For this review, take the finished solid that the model builds, in its own axes (mm). Face numbers are marked on the shaded views. Round coordinates to 2 decimals unless told otherwise and drop trailing zeros. Write each loop counter-clockwise with the first axis right and the second up, starting at its lowest first coordinate (ties: lowest second). Pieces come first, ordered by that corner, then holes. Notation, with made-up numbers: M -37,62 L 10,62 A15 cw 10,68 Z; hole C 5,31 d2. An arc over 180 degrees is marked long. Answer in a Markdown table with one row per item.
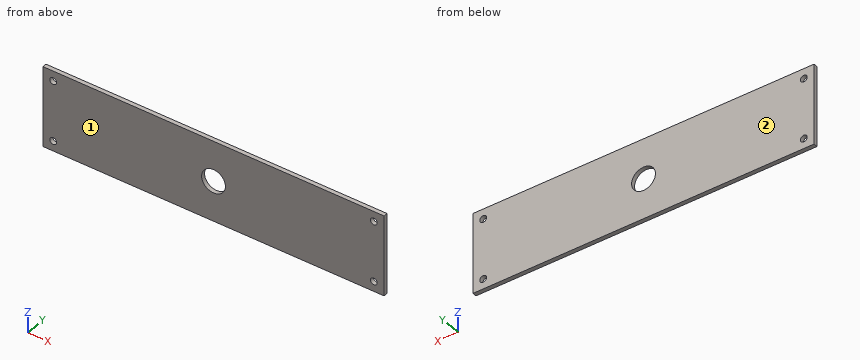
```python
from build123d import *

# Parameters (mm, degrees)
SKETCH1_W           = 500
SKETCH1_H           = 120
SKETCH1_R           = 17.5
SKETCH1_R_2         = 5
BOSS_EXTRUDE1_DEPTH = 3


with BuildPart() as part:
    # Sketch1 → Boss-Extrude1 (new body, symmetric)
    with BuildSketch(Plane(origin=(0, 0, 0), x_dir=(1, 0, 0), z_dir=(0, 1, 0))):
        Rectangle(SKETCH1_W, SKETCH1_H)
        Circle(SKETCH1_R, mode=Mode.SUBTRACT)
        with Locations((-235, 45)):
            Circle(SKETCH1_R_2, mode=Mode.SUBTRACT)
        with Locations((-235, -45)):
            Circle(SKETCH1_R_2, mode=Mode.SUBTRACT)
        with Locations((235, 45)):
            Circle(SKETCH1_R_2, mode=Mode.SUBTRACT)
        with Locations((235, -45)):
            Circle(SKETCH1_R_2, mode=Mode.SUBTRACT)
    extrude(amount=BOSS_EXTRUDE1_DEPTH, both=True)


solid = part.part
```
Q1. Take a section at A-A (y = 0.3). State the section outline as (x, z) points.
Found:
| item | result |
|---|---|
| outline | M -250,-60 L 250,-60 L 250,60 L -250,60 Z; hole C -235,-45 d10; hole C -235,45 d10; hole C 0,0 d35; hole C 235,-45 d10; hole C 235,45 d10 |
Q2. Take a section at C-C (z = 45). State the section outline as (x, y) points, then the cut area to 3 significant figures.
Found:
| item | result |
|---|---|
| outline | M -250,-3 L -240,-3 L -240,3 L -250,3 Z; M -230,-3 L 230,-3 L 230,3 L -230,3 Z; M 240,-3 L 250,-3 L 250,3 L 240,3 Z |
| area | 2,880 mm² |
Q3. Take a section at D-D (x = 0). State the section outline as (y, z) points.
Found:
| item | result |
|---|---|
| outline | M -3,-60 L 3,-60 L 3,-17.5 L -3,-17.5 Z; M -3,17.5 L 3,17.5 L 3,60 L -3,60 Z |
Q4. For probe 1 along X at (y, z) = (-0.5, 45); probe 2 along Z at (x, y) = (235, -1.5); probe 3 along X at (y, z) = (-2.55, -13.5), list the stretches that pass through material, from the lowest coordinate up.
Found:
| item | result |
|---|---|
| probe 1 | -250 to -240, -230 to 230, 240 to 250 |
| probe 2 | -60 to -50, -40 to 40, 50 to 60 |
| probe 3 | -250 to -11.14, 11.14 to 250 |
Q5. Take a section at B-B (x = 235). State the section outline as (y, z) points, then the cut area to 3 significant figures.
Found:
| item | result |
|---|---|
| outline | M -3,-60 L 3,-60 L 3,-50 L -3,-50 Z; M -3,-40 L 3,-40 L 3,40 L -3,40 Z; M -3,50 L 3,50 L 3,60 L -3,60 Z |
| area | 600 mm² |
Q6. Mouldability with a two-part tool opening along Y and no side actions: class the marked faces 1 and 2 as +Y half, -Y half, draft (parallel to the pull), parting line (faces both ways), or undercut.
Found:
| item | result |
|---|---|
| face 1 | -Y half |
| face 2 | +Y half |
